```python
from build123d import *

# Parameters (mm, degrees)
SKETCH1_W            = 155
SKETCH1_H            = 100
BOSS_EXTRUDE1_DEPTH  = 10
SKETCH5_W            = 77
SKETCH5_H            = 50
BOSS_EXTRUDE5_DEPTH  = 200
SKETCH6_W            = 200
SKETCH6_H            = 150
BOSS_EXTRUDE12_DEPTH = 10
BOSS_EXTRUDE13_DEPTH = 10
BOSS_EXTRUDE14_DEPTH = 2.5
MIRROR2_COPY_1_DEPTH = 10
MIRROR2_COPY_2_DEPTH = 2.5
SCALE3_SCALE         = 2


with BuildPart() as part:
    # Sketch1 → Boss-Extrude1 (new body)
    with BuildSketch(Plane.XY):
        Rectangle(SKETCH1_W, SKETCH1_H)
    extrude(amount=BOSS_EXTRUDE1_DEPTH)

    # Sketch5 → Boss-Extrude5 (add)
    with BuildSketch(Plane(origin=(0, 0, 0), x_dir=(-1, 0, 0), z_dir=(0, 0, -1))):
        Rectangle(SKETCH5_W, SKETCH5_H)
    extrude(amount=BOSS_EXTRUDE5_DEPTH)

    # Sketch6 → Boss-Extrude12 (add)
    with BuildSketch(Plane(origin=(0, 0, -200), x_dir=(-1, 0, 0), z_dir=(0, 0, -1))):
        Rectangle(SKETCH6_W, SKETCH6_H)
    extrude(amount=BOSS_EXTRUDE12_DEPTH)

    # Sketch7 → Boss-Extrude13 (add, symmetric)
    with BuildSketch(Plane(origin=(0, 0, 0), x_dir=(0, 0, -1), z_dir=(1, 0, 0))):
        Polygon((1.5, -26.5), (15, -26.5), (15, -25), (0, -25), (0, -35), (1.5, -35), align=None)
    boss_extrude13 = extrude(amount=BOSS_EXTRUDE13_DEPTH, both=True)

    # Sketch7_3 → Boss-Extrude14 (add, symmetric)
    with BuildSketch(Plane(origin=(0, 0, 0), x_dir=(0, 0, -1), z_dir=(1, 0, 0))):
        Polygon((1.5, -31.5), (11.5, -26.5), (1.5, -26.5), align=None)
    boss_extrude14 = extrude(amount=BOSS_EXTRUDE14_DEPTH, both=True)

    # Mirror1: Boss-Extrude13, Boss-Extrude14 across plane
    add(boss_extrude13.mirror(Plane.ZX))
    add(boss_extrude14.mirror(Plane.ZX))

    # Mirror2: Boss-Extrude14, Boss-Extrude13 across plane
    add(boss_extrude14.mirror(Plane(origin=(0, 0, -100), x_dir=(1, 0, 0), z_dir=(0, 0, -1))))
    add(boss_extrude13.mirror(Plane(origin=(0, 0, -100), x_dir=(1, 0, 0), z_dir=(0, 0, -1))))

    # Mirror2 copy 1 sketch → Mirror2 copy 1 (add, symmetric)
    with BuildSketch(Plane(origin=(0, 0, -200), x_dir=(0, 0, 1), z_dir=(1, 0, 0))):
        Polygon((1.5, -26.5), (15, -26.5), (15, -25), (0, -25), (0, -35), (1.5, -35), align=None)
    extrude(amount=MIRROR2_COPY_1_DEPTH, both=True)

    # Mirror2 copy 2 sketch → Mirror2 copy 2 (add, symmetric)
    with BuildSketch(Plane(origin=(0, 0, -200), x_dir=(0, 0, 1), z_dir=(1, 0, 0))):
        Polygon((1.5, -31.5), (11.5, -26.5), (1.5, -26.5), align=None)
    extrude(amount=MIRROR2_COPY_2_DEPTH, both=True)


with BuildPart() as part_1:
    # Scale3: scaled about (0, 0, -112.394978507)
    add(part.part.scale(SCALE3_SCALE).moved(Location((0, 0, 112.394978507))))


solid = part_1.part
```
Read the model definition and answer for the solid it produces. Units are mm, in the model's axes. A direction names the side the tool comes from. Coordinates: 2 decimals unless noted, no trailing zeros. Loops run counter-clockwise (first coordinate to the right, second up) from the corner with the lowest first, then second, coordinate; pieces in that order, holes last.
(1) Flat-ended cylindrical pins translate along their axes: pin 1 Ø6 at (y, z) = (61, -280) entering from -X; pin 2 Ø22 at (y, z) = (-56, 94.5) entering from +X; pin 3 Ø8 at (x, z) = (-4, -175.5) entering from +Y. Find the tip coordinate at first contact, or state that the pin passes through.
Solution:
pin 1: stops at x = -5
pin 2: stops at x = 77
pin 3: stops at y = 50
(2) The part is cut by section D-D (x = -164.5). Determine the outline of the cut face in (y, z), and give its area (3 significant figures).
Solution:
outline: (-150, -307.61) - (150, -307.61) - (150, -287.61) - (-150, -287.61) - close
area: 6,000 mm2
(3) The mould has two halves that part along Z. Classify faces 4 (the face through (-20, 52, -278)), 5 (the face through (-2, 100, 122)), 6 (the face through (3, 2, -307.605)), 7 (the face through (47, -65, -287.605)): released by +Z, released by -Z, zero draft, split by the parting line, or undercut.
Solution:
face 4: undercut
face 5: zero draft
face 6: released by -Z
face 7: undercut
(4) Consider line 1 along Z through (x, y) = (-117, -2); line 2 along Z through (x, y) = (-180, 49); line 3 along Y through (x, z) = (11, -163). Determine where each line is inside the solid, lowest interval first.
Solution:
line 1: z = -307.61 to -287.61, 112.39 to 132.39
line 2: z = -307.61 to -287.61
line 3: y = -50 to 50
(5) The part is cut by section A-A (y = -86). Determine the outline of the cut face in (x, z), and give its area (3 significant figures).
Solution:
outline: (-200, -307.61) - (200, -307.61) - (200, -287.61) - (-200, -287.61) - close; (-155, 112.39) - (155, 112.39) - (155, 132.39) - (-155, 132.39) - close
area: 14,200 mm2
(6) The part is cut by section B-B (x = -85.5). Determine the outline of the cut face in (y, z), and give its area (3 significant figures).
Solution:
outline: (-150, -307.61) - (150, -307.61) - (150, -287.61) - (-150, -287.61) - close; (-100, 112.39) - (100, 112.39) - (100, 132.39) - (-100, 132.39) - close
area: 10,000 mm2
(7) The part is cut by section C-C (y = 8). Determine the outline of the cut face in (x, z), and give its area (3 significant figures).
Solution:
outline: (-200, -307.61) - (200, -307.61) - (200, -287.61) - (77, -287.61) - (77, 112.39) - (155, 112.39) - (155, 132.39) - (-155, 132.39) - (-155, 112.39) - (-77, 112.39) - (-77, -287.61) - (-200, -287.61) - close
area: 75,800 mm2
(8) A tool of negligible diameter and unlimited length cuts with its end or side. For faces 1 (the face through (5, -57, -277)), 2 (the face through (-155, -1, 122)), 3 (the face through (5, 57, -277)), from which of +Z, -Z, +X, -X, +Y, -Y can it reach the whole face along a straight path? Write none if from no direction.
Solution:
face 1: +X, -Y
face 2: +Z, -X, +Y, -Y
face 3: +X, +Y
